Here's the drawing with two shaded views (mm, measured from the low corner). I have some questions. Round coordinates to 2 decimals unless told otherwise and drop trailing zeros. Order: outer loops, then holes, each group sorted by start corner. A loop starts at its lowest first (then second) coordinate and runs counter-clockwise, first axis right, second up. Notation, with made-up numbers: (-6.5, 31) -> (23.5, 31) arc R19 ccw to (23.5, 58) -> close; hole circle Ø9 at (-21.75, 55). An arc over 180 degrees is marked (long way). Answer in a Markdown table with one row per item.
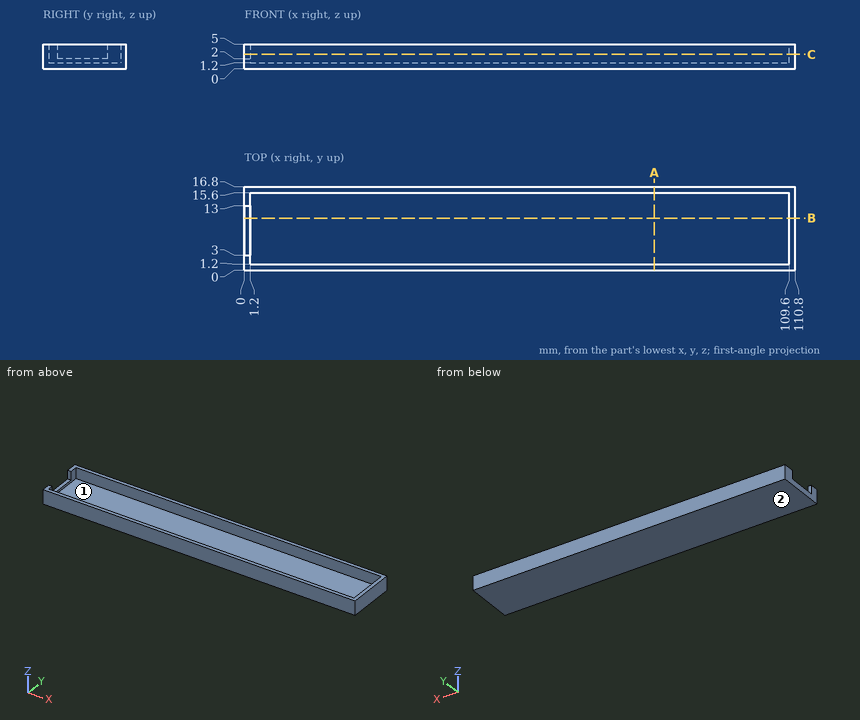
1. Suppose I cut it at B-B on y = 10.5. Write out the boundary of the cut face in (x, z).
Numbers:
| item | result |
|---|---|
| outline | (0, 0) -> (110.8, 0) -> (110.8, 5) -> (109.6, 5) -> (109.6, 1.2) -> (1.2, 1.2) -> (1.2, 2) -> (0, 2) -> close |
2. For pin 1 Ø1.5 at (x, y) = (51, 5) entering from +Z; pin 2 Ø1.3 at (x, y) = (0.5, 7) entering from +Z, each with a flat end and sliding along its axis, tell me the tip position at first contact or that it passes through.
Numbers:
| item | result |
|---|---|
| pin 1 | stops at z = 1.2 |
| pin 2 | stops at z = 2 |
3. Suppose I cut it at C-C on z = 2.9. Write out the boundary of the cut face in (x, y).
Numbers:
| item | result |
|---|---|
| outline | (0, 0) -> (110.8, 0) -> (110.8, 16.8) -> (0, 16.8) -> (0, 13) -> (1.2, 13) -> (1.2, 15.6) -> (109.6, 15.6) -> (109.6, 1.2) -> (1.2, 1.2) -> (1.2, 3) -> (0, 3) -> close |
4. Please list where these lines run through material, in increasing order: line 1 along Y through (x, z) = (30.5, 3.35); line 2 along Z through (x, y) = (27.5, 7.25); line 3 along X through (y, z) = (13.5, 2.55).
Numbers:
| item | result |
|---|---|
| line 1 | y = 0 to 1.2, 15.6 to 16.8 |
| line 2 | z = 0 to 1.2 |
| line 3 | x = 0 to 1.2, 109.6 to 110.8 |
5. Suppose I cut it at A-A on x = 82.5. Write out the boundary of the cut face in (y, z).
Numbers:
| item | result |
|---|---|
| outline | (0, 0) -> (16.8, 0) -> (16.8, 5) -> (15.6, 5) -> (15.6, 1.2) -> (1.2, 1.2) -> (1.2, 5) -> (0, 5) -> close |
6. We'd pull the mould along X, two halves only. Please class the marked faces 1 and 2: released by +X, released by -X, zero draft, split by the parting line, or undercut.
Numbers:
| item | result |
|---|---|
| face 1 | undercut |
| face 2 | zero draft |
